```python
from build123d import *

# Parameters (mm, degrees)
SKETCH1_W                   = 25.4
SKETCH1_H                   = 30.1625
SKETCH1_R                   = 0.762
BOSS_EXTRUDE1_DEPTH         = 3.175
F_1_4_CLEARANCE_HOLE1_D     = 6.5278
F_1_4_CLEARANCE_HOLE1_DEPTH = 6.35
F_1_4_CLEARANCE_HOLE1_TIP   = 1.961148974


with BuildPart() as part:
    # Sketch1 → Boss-Extrude1 (new body)
    with BuildSketch(Plane(origin=(0, 0, 0), x_dir=(1, 0, 0), z_dir=(0, 1, 0))):
        Rectangle(SKETCH1_W, SKETCH1_H)
        with Locations((-7.366, 3.96875)):
            Circle(SKETCH1_R, mode=Mode.SUBTRACT)
        with Locations((-7.366, 10.31875)):
            Circle(SKETCH1_R, mode=Mode.SUBTRACT)
        with BuildLine():
            Line((0, 11.90625), (0, 2.38125))
            ThreePointArc((0, 2.38125), (-1.5875, 0.79375), (-3.175, 2.38125))
            Line((-3.175, 2.38125), (-3.175, 11.90625))
            ThreePointArc((-3.175, 11.90625), (-1.5875, 13.49375), (0, 11.90625))
        make_face(mode=Mode.SUBTRACT)
    extrude(amount=BOSS_EXTRUDE1_DEPTH)

    # 1/4 Clearance Hole1
    with Locations(Plane(origin=(0, 3.175, 0), x_dir=(1, 0, 0), z_dir=(0, 1, 0))):
        with Locations((0, -2.38125)):
            Hole(F_1_4_CLEARANCE_HOLE1_D / 2, depth=F_1_4_CLEARANCE_HOLE1_DEPTH)
            with Locations((0, 0, -(F_1_4_CLEARANCE_HOLE1_DEPTH + F_1_4_CLEARANCE_HOLE1_TIP / 2))):  # 118° drill point
                Cone(0, F_1_4_CLEARANCE_HOLE1_D / 2, F_1_4_CLEARANCE_HOLE1_TIP, mode=Mode.SUBTRACT)


solid = part.part
```
Design review of the part built by this model. Coordinates are the model's own, in mm. A direction names the side the tool comes from. Coordinates: 2 decimals unless noted, no trailing zeros. Loops run counter-clockwise (first coordinate to the right, second up) from the corner with the lowest first, then second, coordinate; pieces in that order, holes last.
Q1. For pin 1 (6 mm diameter, centred on x = 0, z = 2.38, fed in from -Y), flat-tipped, find the tip position at first contact; note if it passes through.
Reported:
pin 1: passes through
Q2. To check wall thickness, follow line 1 (X direction, y = 2, z = -4) (3 decimals); line 2 (X direction, y = 1.2, z = -11.5) (3 decimals); line 3 (X direction, y = 1.25, z = -4.5) (3 decimals). State the ranges of each line that lie inside material, in increasing order.
Reported:
line 1: x = -12.7 to -8.127, -6.605 to -3.175, 0 to 12.7
line 2: x = -12.7 to -3.175, 0 to 12.7
line 3: x = -12.7 to -7.912, -6.82 to -3.175, 0 to 12.7
Q3. The part is to be moulded in two halves that separate along Z. For faces 1 (the face through (-12.7, 2, 0)), 2 (the face through (0, 2, -7)), 3 (the face through (0, 2, -15.081)), say which applies: +Z half, -Z half, draft (parallel to the pull), parting line (faces both ways), or undercut.
Reported:
face 1: draft
face 2: undercut
face 3: -Z half
Q4. Tool access review of faces 4 (the face through (-1.622, 1.565, -13.493)), 5 (the face through (3, 0, 0)): name each direction out of +Z, -Z, +X, -X, +Y, -Y from which nothing blocks a thin tool from reaching the whole face with its end or side.
Reported:
face 4: +Y, -Y
face 5: +Z, -Z, +X, -X, -Y
Q5. We need section A-A on z = -6.5. State the section outline as (x, y) points (3 decimals), and give its area (3 significant figures).
Reported:
outline: (-12.7, 0) - (-3.175, 0) - (-3.175, 3.175) - (-12.7, 3.175) - close; (0, 0) - (12.7, 0) - (12.7, 3.175) - (0, 3.175) - close
area: 70.6 mm2
Q6. We need section B-B on y = 0.4. State the section outline as (x, z) points (1 decimal), and give its area (3 significant figures).
Reported:
outline: (-12.7, -15.1) - (12.7, -15.1) - (12.7, 15.1) - (-12.7, 15.1) - close; hole circle Ø1.5 at (-7.4, -10.3); hole circle Ø1.5 at (-7.4, -4); hole circle Ø6.5 at (0, 2.4); hole (-3.2, -11.9) arc R1.6 ccw to (0, -11.9) - (0, -2.4) arc R1.6 ccw to (-3.2, -2.4) - close
area: 691 mm2
Q7. We need section C-C on z = 1.5. State the section outline as (x, y) points (3 decimals).
Reported:
outline: (-12.7, 0) - (-3.143, 0) - (-3.143, 3.175) - (-12.7, 3.175) - close; (3.143, 0) - (12.7, 0) - (12.7, 3.175) - (3.143, 3.175) - close
